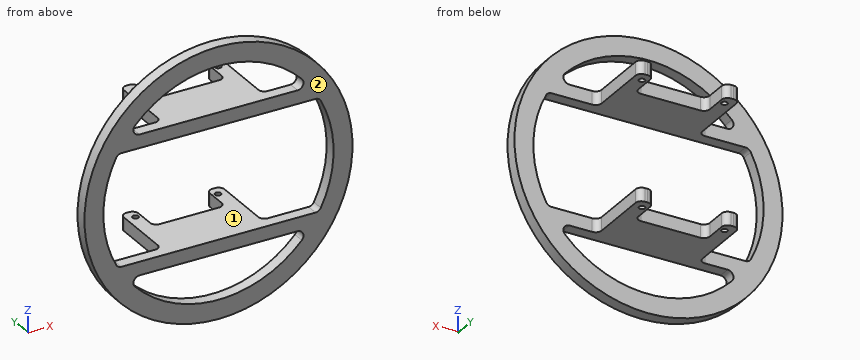
```python
from build123d import *

# Parameters (mm, degrees)
SKETCH1_R           = 1
BOSS_EXTRUDE1_DEPTH = 4.5
SKETCH4_R           = 45
BOSS_EXTRUDE3_DEPTH = 4
FILLET2_R           = 2
FILLET3_R           = 2


with BuildPart() as part:
    # Sketch1 → Boss-Extrude1 (new body)
    with BuildSketch(Plane.XY):
        Polygon((12, 3.5), (16.9, 3.5), (16.9, -20), (-16.9, -20), (-16.9, 3.5), (-12, 3.5), (-12, -7.25), (12, -7.25), align=None)
        with Locations((13.85, 0)):
            Circle(SKETCH1_R, mode=Mode.SUBTRACT)
        with Locations((-13.85, 0)):
            Circle(SKETCH1_R, mode=Mode.SUBTRACT)
    boss_extrude1 = extrude(amount=BOSS_EXTRUDE1_DEPTH)

    # Sketch4 → Boss-Extrude3 (add)
    with BuildSketch(Plane(origin=(0, -20, 0), x_dir=(-1, 0, 0), z_dir=(0, -1, 0))):
        with Locations(Location((0, 18.775, 0), (0, 0, 90))):
            Circle(SKETCH4_R)
        with BuildLine():
            Line((-33.78345564, 0), (33.78345564, 0))
            ThreePointArc((33.78345564, 0), (38.65, 18.775), (33.78345564, 37.55))
            Line((33.78345564, 37.55), (-33.78345564, 37.55))
            ThreePointArc((-33.78345564, 37.55), (-38.65, 18.775), (-33.78345564, 0))
        make_face(mode=Mode.SUBTRACT)
        with BuildLine():
            Line((-30.85606707, -4.5), (30.85606707, -4.5))
            ThreePointArc((30.85606707, -4.5), (0, -19.875), (-30.85606707, -4.5))
        make_face(mode=Mode.SUBTRACT)
        with BuildLine():
            Line((-30.85606707, 42.05), (30.85606707, 42.05))
            ThreePointArc((30.85606707, 42.05), (0, 57.425), (-30.85606707, 42.05))
        make_face(mode=Mode.SUBTRACT)
    extrude(amount=BOSS_EXTRUDE3_DEPTH)

    # Mirror2: Boss-Extrude1 across plane
    add(boss_extrude1.mirror(Plane(origin=(0, 0, -18.775), x_dir=(1, 0, 0), z_dir=(0, 0, -1))))

    # Fillet2
    fillet2_edges = [part.edges().sort_by_distance(p)[0] for p in [
        (-12, -7.25, 2.25),
        (12, -7.25, 2.25),
        (33.78345564, -22, 0),
        (-33.78345564, -22, 0),
        (-33.78345564, -22, -37.55),
        (33.78345564, -22, -37.55),
        (-30.85606707, -22, 4.5),
        (30.85606707, -22, 4.5),
        (30.85606707, -22, -42.05),
        (-30.85606707, -22, -42.05),
        (-12, -7.25, -39.8),
        (12, -7.25, -39.8),
    ]]
    fillet(fillet2_edges, radius=FILLET2_R)

    # Fillet3
    fillet3_edges = [part.edges().sort_by_distance(p)[0] for p in [
        (12, 3.5, 2.25),
        (16.9, 3.5, 2.25),
        (16.9, -20, 2.25),
        (-16.9, -20, 2.25),
        (-16.9, 3.5, 2.25),
        (-12, 3.5, 2.25),
        (-12, 3.5, -39.8),
        (12, 3.5, -39.8),
        (16.9, 3.5, -39.8),
        (16.9, -20, -39.8),
        (-16.9, -20, -39.8),
        (-16.9, 3.5, -39.8),
    ]]
    fillet(fillet3_edges, radius=FILLET3_R)


solid = part.part
```
Here's how the part is built. I have some questions about the finished solid (model axes, mm). Face numbers are marked on the shaded views. Give positions to 0.01 mm unless a question says otherwise; leave off trailing zeros. Order: outer loops, then holes, each group sorted by start corner. A loop starts at its lowest first (then second) coordinate and runs counter-clockwise, first axis right, second up. Notation, with made-up numbers: (3.25, -21) - (57.25, -21) arc R22 cw to (57.25, 11) - close; hole circle Ø5 at (51, 41). An arc over 180 degrees is marked (long way). Answer as a JSON object with one key per item and string values. Group by question number.
Item 1: If we section it at B-B on x = 35.5: Please give me the cut outline in (y, z), and give its area (3 significant figures).
Item 2: If we mould it in two halves opening along Z, with no side actions, what happens to the marked faces 1 and 2? For each: pulls with the +Z half, pulls with the -Z half, needs draft (parallel to the pull), parting line crosses it, or undercut.
Item 3: Please list where these lines run through material, in increasing order: probe 1 along Z at (x, y) = (-22, -20.75); probe 2 along Z at (x, y) = (1, -15.5); probe 3 along Y at (x, z) = (13.85, -40.75).
Item 4: For P1, Ø5, axis at x = -4.5, z = 1.5, coming from the +Y side; P2, Ø5, axis at y = -1.5, z = 2.5, coming from the -X side; P3, Ø3, axis at x = 13.85, y = 0, coming from the -Z side, each with a flat end and sliding along its axis, tell me the tip position at first contact or that it passes through.
Item 5: If we section it at A-A on y = -12.25: Please give me the cut outline in (x, z), and give its area (3 significant figures).
Result set:
{
 "1": {"outline": "(-24, -46.43) - (-20, -46.43) - (-20, -34.06) - (-24, -34.06) - close; (-24, -3.49) - (-20, -3.49) - (-20, 8.88) - (-24, 8.88) - close", "area": "99.0 mm²"},
 "2": {"face 1": "undercut", "face 2": "needs draft"},
 "3": {"probe 1": "-58.03 to -50.55, -42.05 to -37.55, 0 to 4.5, 13 to 20.48", "probe 2": "-42.05 to -37.55, 0 to 4.5", "probe 3": "-24 to -1, 1 to 3.49"},
 "4": {"P1": "y = -7.25", "P2": "x = -16.9", "P3": "z = -42.05"},
 "5": {"outline": "(-16.9, -42.05) - (16.9, -42.05) - (16.9, -37.55) - (-16.9, -37.55) - close; (-16.9, 0) - (16.9, 0) - (16.9, 4.5) - (-16.9, 4.5) - close", "area": "304 mm²"}
}
